Build history of the part. All positions in model axes, mm. A direction names the side the tool comes from. Round coordinates to 2 decimals unless told otherwise and drop trailing zeros. Order: outer loops, then holes, each group sorted by start corner. A loop starts at its lowest first (then second) coordinate and runs counter-clockwise, first axis right, second up. Notation, with made-up numbers: (4.5, -12) -> (27.5, -12) arc R21 cw to (27.5, 27) -> close; hole circle Ø11 at (66, -24.5). An arc over 180 degrees is marked (long way). Write item = value, one per line.
from build123d import *

# Parameters (mm, degrees)
SKETCH1_R                    = 18.4
BOSS_EXTRUDE1_DEPTH          = 20
SKETCH2_R                    = 17.4
BOSS_EXTRUDE2_DEPTH          = 30
SKETCH3_R                    = 6
BOSS_EXTRUDE3_DEPTH          = 6.5
FILLET1_R                    = 0.5
SKETCH4_R                    = 3
BOSS_EXTRUDE4_DEPTH          = 15.5
CUT_EXTRUDE1_START           = -12
CUT_EXTRUDE1_DEPTH           = 12
F_3_0_3_DIAMETER_HOLE1_D     = 3
F_3_0_3_DIAMETER_HOLE1_DEPTH = 3
F_3_0_3_DIAMETER_HOLE1_TIP   = 0.901290929
CUT_EXTRUDE2_DEPTH           = 1
SKETCH9_R                    = 4
BOSS_EXTRUDE5_DEPTH          = 1
FILLET2_R                    = 0.5
SKETCH11_W                   = 3.5
SKETCH11_H                   = 1
BOSS_EXTRUDE7_DEPTH          = 5.6
FILLET3_R                    = 0.5
SKETCH14_R                   = 1.5
BOSS_EXTRUDE9_DEPTH          = 8.55
FILLET4_R                    = 0.5


with BuildPart() as part:
    # Sketch1 → Boss-Extrude1 (new body)
    with BuildSketch(Plane.XY):
        Circle(SKETCH1_R)
    extrude(amount=BOSS_EXTRUDE1_DEPTH)

    # Sketch2 → Boss-Extrude2 (add)
    with BuildSketch(Plane(origin=(0, 0, 0), x_dir=(-1, 0, 0), z_dir=(0, 0, -1))):
        with Locations(Location((0, 0, 0), (0, 0, 180))):
            Circle(SKETCH2_R)
    extrude(amount=BOSS_EXTRUDE2_DEPTH)

    # Sketch3 → Boss-Extrude3 (add)
    with BuildSketch(Plane.XY.offset(20)):
        with Locations(Location((7, 0, 0), (0, 0, 180))):
            Circle(SKETCH3_R)
    extrude(amount=BOSS_EXTRUDE3_DEPTH)

    # Fillet1
    fillet1_edges = [part.edges().sort_by_distance(p)[0] for p in [
        (13, 0, 26.5),
    ]]
    fillet(fillet1_edges, radius=FILLET1_R)

    # Sketch4 → Boss-Extrude4 (add)
    with BuildSketch(Plane.XY.offset(26.5)):
        with Locations((7, 0)):
            Circle(SKETCH4_R)
    extrude(amount=BOSS_EXTRUDE4_DEPTH)

    # Sketch5 → Cut-Extrude1 (cut)
    with BuildSketch(Plane.XY.offset(42).offset(CUT_EXTRUDE1_START)):
        with BuildLine():
            Line((5.503337045, 2.6), (8.496662955, 2.6))
            ThreePointArc((8.496662955, 2.6), (7, 3), (5.503337045, 2.6))
        make_face()
    extrude(amount=CUT_EXTRUDE1_DEPTH, mode=Mode.SUBTRACT)

    # Ø3.0 (3) Diameter Hole1
    with Locations(Plane.XY.offset(20)):
        with Locations((-13.423393759, 7.75), (-13.423393759, -7.75), (0, -15.5), (13.423393759, 7.75), (0, 15.5), (13.423393759, -7.75)):
            Hole(F_3_0_3_DIAMETER_HOLE1_D / 2, depth=F_3_0_3_DIAMETER_HOLE1_DEPTH)
            with Locations((0, 0, -(F_3_0_3_DIAMETER_HOLE1_DEPTH + F_3_0_3_DIAMETER_HOLE1_TIP / 2))):  # 118° drill point
                Cone(0, F_3_0_3_DIAMETER_HOLE1_D / 2, F_3_0_3_DIAMETER_HOLE1_TIP, mode=Mode.SUBTRACT)

    # Sketch8 → Cut-Extrude2 (cut)
    with BuildSketch(Plane.XY.offset(20)):
        with BuildLine():
            ThreePointArc((10.116155685, 7.342574083), (-12.5, 0), (10.116155685, -7.342574083))
            ThreePointArc((10.116155685, -7.342574083), (-1.05978604, 0), (10.116155685, 7.342574083))
        make_face()
    extrude(amount=-CUT_EXTRUDE2_DEPTH, mode=Mode.SUBTRACT)

    # Sketch9 → Boss-Extrude5 (add)
    with BuildSketch(Plane(origin=(0, 0, -30), x_dir=(-1, 0, 0), z_dir=(0, 0, -1))):
        Circle(SKETCH9_R)
    extrude(amount=BOSS_EXTRUDE5_DEPTH)

    # Fillet2
    fillet2_edges = [part.edges().sort_by_distance(p)[0] for p in [
        (4, 0, -31),
    ]]
    fillet(fillet2_edges, radius=FILLET2_R)

    # Sketch11 → Boss-Extrude7 (add)
    with BuildSketch(Plane(origin=(0, 0, -30), x_dir=(-1, 0, 0), z_dir=(0, 0, -1))):
        with Locations((0, 12.05)):
            Rectangle(SKETCH11_W, SKETCH11_H)
        with Locations((0, -12.05)):
            Rectangle(SKETCH11_W, SKETCH11_H)
    extrude(amount=BOSS_EXTRUDE7_DEPTH)

    # Fillet3
    fillet3_edges = [part.edges().sort_by_distance(p)[0] for p in [
        (1.75, 12.05, -35.6),
        (-1.75, 12.05, -35.6),
        (-1.75, -12.05, -35.6),
        (1.75, -12.05, -35.6),
    ]]
    fillet(fillet3_edges, radius=FILLET3_R)

    # Sketch14 → Boss-Extrude9 (add)
    with BuildSketch(Plane(origin=(0, 0, -31), x_dir=(-1, 0, 0), z_dir=(0, 0, -1))):
        Circle(SKETCH14_R)
    extrude(amount=BOSS_EXTRUDE9_DEPTH)

    # Fillet4
    # the kernel refuses this fillet: 0.5 mm, written as the material it takes off along each edge
    with BuildSketch(Plane(origin=(7, 0, 42), x_dir=(0.4622655728594592, 0.8867415295050277, 0), z_dir=(0.8867415295050277, -0.4622655728594592, 0))) as fillet4_piece_1:
        with BuildLine():
            CenterArc((3 - FILLET4_R, -FILLET4_R), FILLET4_R, 0, 90)
            Line((3 - FILLET4_R, 0), (3 - FILLET4_R, FILLET4_R * 0.02))
            Line((3 - FILLET4_R, FILLET4_R * 0.02), (3 + FILLET4_R * 0.02, FILLET4_R * 0.02))
            Line((3 + FILLET4_R * 0.02, FILLET4_R * 0.02), (3 + FILLET4_R * 0.02, -FILLET4_R))
            Line((3 + FILLET4_R * 0.02, -FILLET4_R), (3, -FILLET4_R))
        make_face()
    revolve(axis=Axis((7, 0, 42), (0, 0, 1)), revolution_arc=297.533397677, mode=Mode.SUBTRACT)
    with BuildSketch(Plane(origin=(7, 0, 42), x_dir=(1, 0, 0), z_dir=(0, -1, 0))) as fillet4_piece_2:
        with BuildLine():
            CenterArc((3 - FILLET4_R, -FILLET4_R), FILLET4_R, 0, 90)
            Line((3 - FILLET4_R, 0), (3 - FILLET4_R, FILLET4_R * 0.02))
            Line((3 - FILLET4_R, FILLET4_R * 0.02), (3 + FILLET4_R * 0.02, FILLET4_R * 0.02))
            Line((3 + FILLET4_R * 0.02, FILLET4_R * 0.02), (3 + FILLET4_R * 0.02, -FILLET4_R))
            Line((3 + FILLET4_R * 0.02, -FILLET4_R), (3, -FILLET4_R))
        make_face()
    revolve(axis=Axis((7, 0, 42), (0, 0, 1)), revolution_arc=117.379597562, mode=Mode.SUBTRACT)


solid = part.part
Q1. Cut at C-C, the plane x = -7. List the corners of the cut face in (y, z), and give its area (3 significant figures).
Check values:
outline = (-17.02, 0) -> (-15.93, 0) -> (-15.93, -30) -> (15.93, -30) -> (15.93, 0) -> (17.02, 0) -> (17.02, 20) -> (10.36, 20) -> (10.36, 19) -> (-10.36, 19) -> (-10.36, 20) -> (-17.02, 20) -> close
area = 1,620 mm²
Q2. Cut at D-D, the plane z = 4. List the corners of the cut face in (x, y), and give its area (3 significant figures).
Check values:
outline = circle Ø36.8 at (0, 0)
area = 1,060 mm²
Q3. Probe probe 1 along Y at (x, z) = (0, 18.75); probe 2 along X at (y, z) = (7.75, 18.5); probe 3 along Y at (x, z) = (-14, 17.5). List the from-to ranges inside material, lowest first.
Check values:
probe_1 = -18.4 to -17, -14 to 14, 17 to 18.4
probe_2 = -16.69 to -14.92, -11.92 to 11.92, 14.92 to 16.69
probe_3 = -11.94 to -9.13, -6.37 to 6.37, 9.13 to 11.94
Q4. Flat gauge pins, fed straight in: pin 1 (10.5 mm diameter, centred on x = -2.5, y = -5.5, fed in from -Z); pin 2 (4 mm diameter, centred on x = -13.42, y = 7.75, fed in from +Z); pin 3 (6 mm diameter, centred on x = 1, z = -5.5, fed in from +Y); pin 4 (0.5 mm diameter, centred on y = 12, z = -33, fed in from -X). Where does each tip first touch, or does it go through?
Check values:
pin_1 = -39.55
pin_2 = 20
pin_3 = 17.4
pin_4 = -1.75
Q5. Cut at A-A, the plane z = -33. List the corners of the cut face in (x, y).
Check values:
outline = (-1.75, -12.55) -> (1.75, -12.55) -> (1.75, -11.55) -> (-1.75, -11.55) -> close; (-1.75, 11.55) -> (1.75, 11.55) -> (1.75, 12.55) -> (-1.75, 12.55) -> close; circle Ø3 at (0, 0)
Q6. Which spindle directions (+Z, -Z, +X, -X, +Y, -Y) get a long thin tool onto all of the face, cutting with end or side? Do faces 1 (the face through (0, 11.55, -33)), 2 (the face through (-14.6, -11.2, 9.9)), 3 (the face through (0, 0, 20)), 4 (the face through (0.867, -3.905, -30.246)). Say none if no direction does.
Check values:
face_1 = -Z, +X, -X
face_2 = +Z, -Z
face_3 = +Z
face_4 = -Z
Q7. Mould opens along Y. For faces 5 (the face through (-3.772, 16.986, -14.79)), 6 (the face through (0, 12.55, -33)), 7 (the face through (-1.057, -0.222, 19.507)) say: released by +Y, released by -Y, zero draft, split by the parting line, or undercut.
Check values:
face_5 = split by the parting line
face_6 = released by +Y
face_7 = undercut
